Part model, mm, in its own coordinate system. A direction names the side the tool comes from. Give positions to 0.01 mm unless a question says otherwise; leave off trailing zeros. Order: outer loops, then holes, each group sorted by start corner. A loop starts at its lowest first (then second) coordinate and runs counter-clockwise, first axis right, second up. Notation, with made-up numbers: (52.25, -20.75) - (67.25, -20.75) arc R17 ccw to (67.25, -7.75) - close; hole circle Ø8 at (75.5, -28.75). An arc over 180 degrees is marked (long way). One line per item, written item: value.
```python
from build123d import *

# Parameters (mm, degrees)
SKETCH1_R               = 16.25
BOSS_EXTRUDE1_DEPTH     = 10
BOSS_EXTRUDE2_START     = 3.1
SKETCH1_3_R             = 16.25
BOSS_EXTRUDE2_DEPTH     = 6.9
BOSS_EXTRUDE3_START     = 3.1
SKETCH1_4_R             = 2.05
BOSS_EXTRUDE3_DEPTH     = 3.1
SKETCH2_R               = 1.5
CUT_EXTRUDE1_DEPTH      = 1
CUT_EXTRUDE1_DEPTH_BACK = 11
BOSS_EXTRUDE4_DEPTH     = 5
SKETCH3_R               = 5
CUT_EXTRUDE2_DEPTH      = 11.134556711
CUT_EXTRUDE2_DEPTH_BACK = 54.505053596


with BuildPart() as part:
    # Sketch1 → Boss-Extrude1 (new body)
    with BuildSketch(Plane(origin=(0, 0, 0), x_dir=(0, 1, 0), z_dir=(0, 0, 1))):
        with BuildLine():
            Line((21.213203436, -21.213203436), (22.455838333, -1.409015532))
            ThreePointArc((22.455838333, -1.409015532), (-15.909902577, 15.909902577), (1.409015532, -22.455838333))
            Line((1.409015532, -22.455838333), (21.213203436, -21.213203436))
        make_face()
        Circle(SKETCH1_R, mode=Mode.SUBTRACT)
    extrude(amount=BOSS_EXTRUDE1_DEPTH)

    # Sketch1<3> → Boss-Extrude2 (add)
    with BuildSketch(Plane(origin=(0, 0, 0), x_dir=(0, 1, 0), z_dir=(0, 0, 1)).offset(BOSS_EXTRUDE2_START)):
        Circle(SKETCH1_3_R)
        Polygon((-3.5, 9.979274058), (0, 7.958548116), (3.5, 9.979274058), (3.5, 14.020725942), (0, 16.041451884), (-3.5, 14.020725942), align=None, mode=Mode.SUBTRACT)
        Polygon((9.979274058, 3.5), (7.958548116, 0), (9.979274058, -3.5), (14.020725942, -3.5), (16.041451884, 0), (14.020725942, 3.5), align=None, mode=Mode.SUBTRACT)
        Polygon((3.5, -9.979274058), (0, -7.958548116), (-3.5, -9.979274058), (-3.5, -14.020725942), (0, -16.041451884), (3.5, -14.020725942), align=None, mode=Mode.SUBTRACT)
        Polygon((-9.979274058, -3.5), (-7.958548116, 0), (-9.979274058, 3.5), (-14.020725942, 3.5), (-16.041451884, 0), (-14.020725942, -3.5), align=None, mode=Mode.SUBTRACT)
    extrude(amount=BOSS_EXTRUDE2_DEPTH)

    # Sketch1<4> → Boss-Extrude3 (add)
    with BuildSketch(Plane(origin=(0, 0, 0), x_dir=(0, 1, 0), z_dir=(0, 0, 1)).offset(BOSS_EXTRUDE3_START)):
        Polygon((3.5, -14.020725942), (3.5, -9.979274058), (0, -7.958548116), (-3.5, -9.979274058), (-3.5, -14.020725942), (0, -16.041451884), align=None)
        with Locations((0, -12)):
            Circle(SKETCH1_4_R, mode=Mode.SUBTRACT)
        Polygon((14.020725942, 3.5), (9.979274058, 3.5), (7.958548116, 0), (9.979274058, -3.5), (14.020725942, -3.5), (16.041451884, 0), align=None)
        with Locations((12, 0)):
            Circle(SKETCH1_4_R, mode=Mode.SUBTRACT)
        Polygon((-3.5, 14.020725942), (-3.5, 9.979274058), (0, 7.958548116), (3.5, 9.979274058), (3.5, 14.020725942), (0, 16.041451884), align=None)
        with Locations((0, 12)):
            Circle(SKETCH1_4_R, mode=Mode.SUBTRACT)
        Polygon((-14.020725942, -3.5), (-9.979274058, -3.5), (-7.958548116, 0), (-9.979274058, 3.5), (-14.020725942, 3.5), (-16.041451884, 0), align=None)
        with Locations((-12, 0)):
            Circle(SKETCH1_4_R, mode=Mode.SUBTRACT)
    extrude(amount=BOSS_EXTRUDE3_DEPTH)

    # Sketch2 → Cut-Extrude1 (cut, two sides)
    with BuildSketch(Plane.XY.offset(10)) as cut_extrude1_sk:
        with Locations((8.838834765, -8.838834765)):
            Circle(SKETCH2_R)
        with Locations((-8.838834765, 8.838834765)):
            Circle(SKETCH2_R)
    extrude(amount=CUT_EXTRUDE1_DEPTH, mode=Mode.SUBTRACT)
    extrude(cut_extrude1_sk.sketch, amount=-CUT_EXTRUDE1_DEPTH_BACK, mode=Mode.SUBTRACT)

    # Sketch2<3> → Boss-Extrude4 (add)
    with BuildSketch(Plane.XY.offset(10)):
        Polygon((-5.224829065, -12.295896877), (-12.295896877, -5.224829065), (-18.869320131, -11.798252319), (-11.798252319, -18.869320131), align=None)
        Polygon((-12.295896877, -5.224829065), (-13.003003658, -4.517722284), (-19.576426912, -11.091145538), (-18.869320131, -11.798252319), align=None)
        Polygon((-4.517722284, -13.003003658), (-5.224829065, -12.295896877), (-11.798252319, -18.869320131), (-11.091145538, -19.576426912), align=None)
        Polygon((6.775170935, -0.295896877), (-0.295896877, 6.775170935), (-6.775170935, 0.295896877), (0.295896877, -6.775170935), align=None)
        Polygon((-0.295896877, 6.775170935), (-1.003003658, 7.482277716), (-7.482277716, 1.003003658), (-6.775170935, 0.295896877), align=None)
        Polygon((7.482277716, -1.003003658), (6.775170935, -0.295896877), (0.295896877, -6.775170935), (1.003003658, -7.482277716), align=None)
        Polygon((19.576426912, 11.091145538), (18.869320131, 11.798252319), (12.295896877, 5.224829065), (13.003003658, 4.517722284), align=None)
        Polygon((18.869320131, 11.798252319), (11.798252319, 18.869320131), (5.224829065, 12.295896877), (12.295896877, 5.224829065), align=None)
        Polygon((11.798252319, 18.869320131), (11.091145538, 19.576426912), (4.517722284, 13.003003658), (5.224829065, 12.295896877), align=None)
    extrude(amount=BOSS_EXTRUDE4_DEPTH)

    # Sketch3 → Cut-Extrude2 (cut, two sides)
    with BuildSketch(Plane(origin=(-15.333786225, -15.333786225, 0), x_dir=(0.707106781, -0.707106781, 0), z_dir=(-0.707106781, -0.707106781, 0))) as cut_extrude2_sk:
        with Locations((0, 15)):
            Circle(SKETCH3_R)
    extrude(amount=CUT_EXTRUDE2_DEPTH, mode=Mode.SUBTRACT)
    extrude(cut_extrude2_sk.sketch, amount=-CUT_EXTRUDE2_DEPTH_BACK, mode=Mode.SUBTRACT)


solid = part.part
```
1) Mould opens along X. For faces 5 (the flat face through (16, 8, 15)), 6 (the flat face through (-11.97, -5.55, 11.75)), 7 (the flat face through (7.85, 16.336, 12.465)), 8 (the flat face through (-2, 14, 6.2)) say: released by +X, released by -X, zero draft, split by the parting line, or undercut.
Outcome:
face 5: zero draft
face 6: undercut
face 7: released by -X
face 8: undercut
2) Drill centre lines: line 1 along Y through (x, z) = (0, 4.5); line 2 along X through (y, z) = (0, 7.75); line 3 along X through (y, z) = (-7, 11.75). Where is each one in solid material? Low to high. Write a range as from..to.
Outcome:
line 1: y = -22.5..-14.05, -9.95..9.95, 14.05..22.5
line 2: x = -22.5..-16.04, -7.96..7.96, 16.04..22.5
line 3: x = -15.49..-12.37, 0.52..1.49
3) Pin check, flat tips, straight feed: pin 1 (4 mm diameter, centred on y = 8.5, z = 7.5, fed in from +X); pin 2 (4 mm diameter, centred on x = -12, z = 7.5, fed in from +Y); pin 3 (4 mm diameter, centred on y = -5, z = 7.5, fed in from -X); pin 4 (7.5 mm diameter, centred on x = -10.5, y = 1, fed in from +Z). Stop position of each tip, or through.
Outcome:
pin 1: stops at x = 22.14
pin 2: stops at y = 20.16
pin 3: stops at x = -22.3
pin 4: stops at z = 15
4) Which spindle directions (+Z, -Z, +X, -X, +Y, -Y) get a long thin tool onto all of the face, cutting with end or side? Do faces 1 (the flat face through (-4.197, 4.288, 12.465)), 2 (the flat face through (11.97, 5.55, 11.75)), 3 (the flat face through (-1.8, 9, 8.1)), 4 (the flat face through (-4, 4, 15)). Say none if no direction does.
Outcome:
face 1: +Z, -X, +Y
face 2: +Z, -Y
face 3: +Z
face 4: +Z, +X, -X, +Y, -Y
5) Cut at B-B, the plane z = 3.75. Give the cut face in (x, y), then the cut area to 3 significant figures.
Outcome:
outline: (1.41, 22.46) arc R22.5 ccw (long way) to (22.46, 1.41) - (21.21, 21.21) - close; hole circle Ø4.1 at (-12, 0); hole circle Ø3 at (-8.84, 8.84); hole circle Ø4.1 at (0, -12); hole circle Ø4.1 at (0, 12); hole circle Ø3 at (8.84, -8.84); hole circle Ø4.1 at (12, 0)
area: 1,600 mm^2
6) Cut at A-A, the plane z = 12.5. Give the cut face in (x, y), then the cut area to 3 significant figures.
Outcome:
outline: (-19.58, -11.09) - (-18.4, -12.27) - (-11.82, -5.7) - (-13, -4.52) - close; (-12.27, -18.4) - (-11.09, -19.58) - (-4.52, -13) - (-5.7, -11.82) - close; (-7.48, 1) - (-6.3, -0.18) - (0.18, 6.3) - (-1, 7.48) - close; (-0.18, -6.3) - (1, -7.48) - (7.48, -1) - (6.3, 0.18) - close; (4.52, 13) - (5.7, 11.82) - (12.27, 18.4) - (11.09, 19.58) - close; (11.82, 5.7) - (13, 4.52) - (19.58, 11.09) - (18.4, 12.27) - close
area: 92.7 mm^2
